Here's the drawing with two shaded views (mm, measured from the low corner). I have some questions. Coordinates: 2 decimals unless noted, no trailing zeros. Write each loop counter-clockwise with the first axis right and the second up, starting at its lowest first coordinate (ties: lowest second). Pieces come first, ordered by that corner, then holes.
Item 1: If we section it at A-A (z = 4.5): Please give me the cut outline in (x, y), then the cut area to 3 significant figures.
Item 2: If I drill on line 1 (X direction, y = 7.5, z = 17); line 2 (Y direction, x = 15, z = 11); line 3 (X direction, y = 57.5, z = 5.75), over which ranges is the centre line in solid material (lowest first)?
Item 3: If we section it at B-B (y = 57.5): Please give me the cut outline in (x, z), then the cut area to 3 significant figures.
Item 4: If we section it at C-C (x = 90): Please give me the cut outline in (y, z).
Item 5: I'm going to push flat-ended pins straight in: pin 1 Ø10 at (y, z) = (27, 7.5) entering from -X; pin 2 Ø7.5 at (x, y) = (90, 7.5) entering from +Z; pin 3 Ø5 at (x, y) = (90, 57.5) entering from -Z. Where does each tip first touch, or does it pass through?
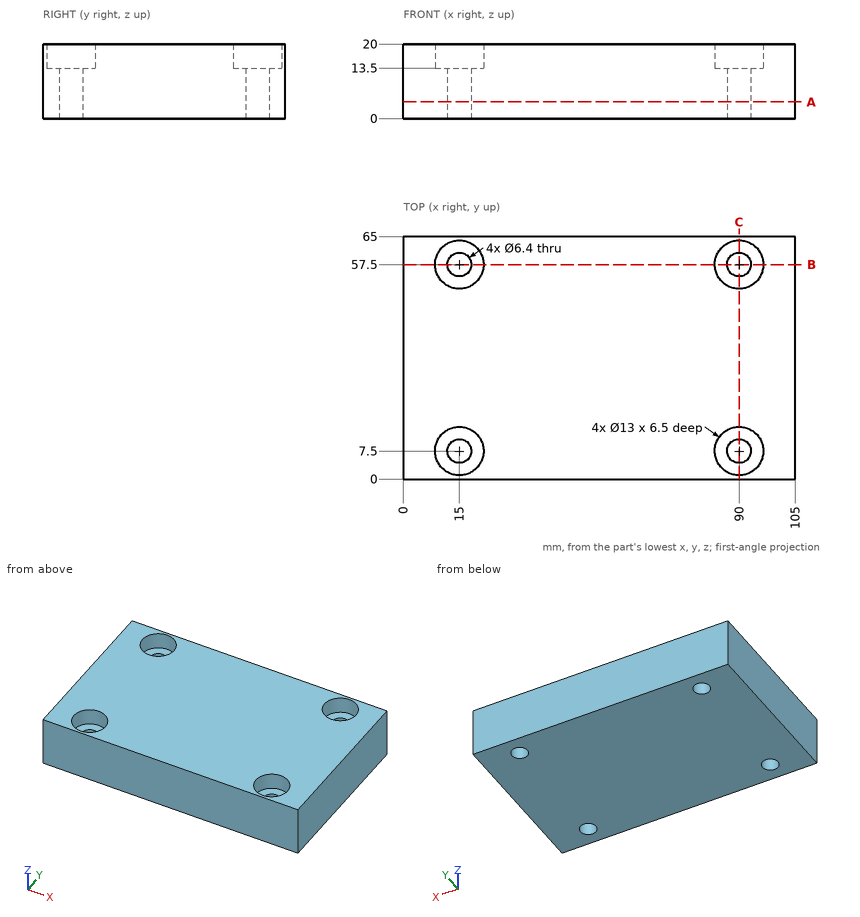
Answer list:
1. outline: (0, 0) - (105, 0) - (105, 65) - (0, 65) - close; hole circle Ø6.4 at (15, 7.5); hole circle Ø6.4 at (15, 57.5); hole circle Ø6.4 at (90, 7.5); hole circle Ø6.4 at (90, 57.5)
1. area: 6,700 mm2
2. line 1: x = 0 to 8.5, 21.5 to 83.5, 96.5 to 105
2. line 2: y = 0 to 4.3, 10.7 to 54.3, 60.7 to 65
2. line 3: x = 0 to 11.8, 18.2 to 86.8, 93.2 to 105
3. outline: (0, 0) - (11.8, 0) - (11.8, 13.5) - (8.5, 13.5) - (8.5, 20) - (0, 20) - close; (18.2, 0) - (86.8, 0) - (86.8, 13.5) - (83.5, 13.5) - (83.5, 20) - (21.5, 20) - (21.5, 13.5) - (18.2, 13.5) - close; (93.2, 0) - (105, 0) - (105, 20) - (96.5, 20) - (96.5, 13.5) - (93.2, 13.5) - close
3. area: 1,760 mm2
4. outline: (0, 0) - (4.3, 0) - (4.3, 13.5) - (1, 13.5) - (1, 20) - (0, 20) - close; (10.7, 0) - (54.3, 0) - (54.3, 13.5) - (51, 13.5) - (51, 20) - (14, 20) - (14, 13.5) - (10.7, 13.5) - close; (60.7, 0) - (65, 0) - (65, 20) - (64, 20) - (64, 13.5) - (60.7, 13.5) - close
5. pin 1: stops at x = 0
5. pin 2: stops at z = 13.5
5. pin 3: passes through
